from build123d import *

# Parameters (mm, degrees)
F0_R     = 95.2277676599
F1_DEPTH = 50
F2_R     = 14.1001536821
F3_DEPTH = 100
F4_DEPTH = 200
F6_D     = 5


with BuildPart() as f1:
    # F0 (on Front) → F1 (new body)
    with BuildSketch(Plane.XZ):
        Circle(F0_R)
    extrude(amount=F1_DEPTH)

    # F2 (on face) → F3 (join)
    with BuildSketch(Plane.XZ.offset(50)):
        Circle(F2_R)
    extrude(amount=F3_DEPTH)

    # F4 (add): a face of the model
    f4_faces = [f1.faces().sort_by_distance(p)[0] for p in [
        (0, 0, 0),
    ]]
    extrude(f4_faces, amount=F4_DEPTH)

    # F6 (through all)
    with Locations(Plane.XZ.offset(150)):
        with Locations((0, 0)):
            Hole(F6_D / 2)


solid = f1.part
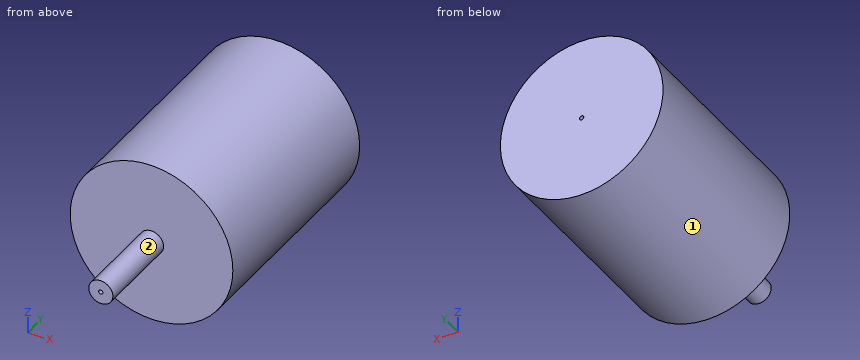
Could you check a few things on this model? Use its own coordinates, in mm. Face numbers are marked on the shaded views. A direction names the side the tool comes from. Round coordinates to 2 decimals unless told otherwise and drop trailing zeros. Write each loop counter-clockwise with the first axis right and the second up, starting at its lowest first coordinate (ties: lowest second). Pieces come first, ordered by that corner, then holes. Notation, with made-up numbers: (78.25, 2.25) -> (119.25, 2.25) arc R13 cw to (119.25, 27.25) -> close; hole circle Ø9 at (-18.5, 52). An arc over 180 degrees is marked (long way). Use a Markdown table: item, result.
1. Please list where these lines run through material, in increasing order: probe 1 along Z at (x, y) = (0, 76); probe 2 along Z at (x, y) = (0, -64); probe 3 along Y at (x, z) = (63, -3).
Answer key:
| item | result |
|---|---|
| probe 1 | z = -95.23 to -2.5, 2.5 to 95.23 |
| probe 2 | z = -14.1 to -2.5, 2.5 to 14.1 |
| probe 3 | y = -50 to 200 |
2. Which directions (+Z, -Z, +X, -X, +Y, -Y) give clear straight access to the entire face, cutting with the end or side of a thin tool? Please do the marked faces 1 and 2.
Answer key:
| item | result |
|---|---|
| face 1 | +Y, -Y |
| face 2 | -Y |
3. If we section it at D-D (y = 125): List the corners of the cut face in (x, z) for me.
Answer key:
| item | result |
|---|---|
| outline | circle Ø190.46 at (0, 0); hole circle Ø5 at (0, 0) |
4. If we section it at B-B (z = 34.5): List the corners of the cut face in (x, y) for me.
Answer key:
| item | result |
|---|---|
| outline | (-88.76, -50) -> (88.76, -50) -> (88.76, 200) -> (-88.76, 200) -> close |
5. For pin 1 Ø2 at (x, y) = (68.5, -0.5) entering from +Z; pin 2 Ø6 at (x, y) = (35, 27) entering from +Z; pin 3 Ø4 at (x, z) = (0, 0) entering from +Y; pin 4 Ø1.5 at (x, y) = (-3, -2.5) entering from +Z, each with a flat end and sliding along its axis, tell me the tip position at first contact or that it passes through.
Answer key:
| item | result |
|---|---|
| pin 1 | stops at z = 67.17 |
| pin 2 | stops at z = 89.69 |
| pin 3 | passes through |
| pin 4 | stops at z = 95.2 |
6. If we section it at A-A (y = -96.5): List the corners of the cut face in (x, z) for me, then the cut area to 3 significant figures.
Answer key:
| item | result |
|---|---|
| outline | circle Ø28.2 at (0, 0); hole circle Ø5 at (0, 0) |
| area | 605 mm^2 |
7. If we section it at C-C (x = 81.5): List the corners of the cut face in (y, z) for me, then the cut area to 3 significant figures.
Answer key:
| item | result |
|---|---|
| outline | (-50, -49.26) -> (200, -49.26) -> (200, 49.26) -> (-50, 49.26) -> close |
| area | 24,600 mm^2 |
